Geometry check sheet. Reference: the model listing, model coordinates, mm. Face numbers are marked on the shaded views. A direction names the side the tool comes from. Round coordinates to 2 decimals unless told otherwise and drop trailing zeros. Loops run counter-clockwise (first coordinate to the right, second up) from the corner with the lowest first, then second, coordinate; pieces in that order, holes last. Notation, with made-up numbers: (-12.75, 62.5) -> (37.25, 62.5) arc R23 cw to (37.25, 98.5) -> close; hole circle Ø2 at (15, 18). An arc over 180 degrees is marked (long way). Use one line per item in the form item = value.
from build123d import *

# Parameters (mm, degrees)
SKETCH_1_W          = 39.5
SKETCH_1_H          = 34.04
EXTRUDE_1_DEPTH     = 2
SKETCH_2_R          = 1.25
CUT_EXTRUDE_1_DEPTH = 2
SKETCH_3_R          = 12.5
EXTRUDE_2_DEPTH     = 5
FILLET_1_R          = 1
SKETCH_4_W          = 8
SKETCH_4_H          = 8.5
SKETCH_4_H_2        = 12
EXTRUDE_3_DEPTH     = 5
SKETCH_5_R          = 1
CUT_EXTRUDE_2_DEPTH = 5


with BuildPart() as part:
    # 草图1 → 凸台-拉伸1 (new body)
    with BuildSketch(Plane.XY):
        Rectangle(SKETCH_1_W, SKETCH_1_H)
    extrude(amount=EXTRUDE_1_DEPTH)

    # 草图2 → 切除-拉伸1 (cut)
    with BuildSketch(Plane.XY.offset(2)):
        with Locations((-16.95, 14.225)):
            Circle(SKETCH_2_R)
        with Locations((-16.95, -14.225)):
            Circle(SKETCH_2_R)
        with Locations((8.07, 14.225)):
            Circle(SKETCH_2_R)
        with Locations((8.07, -14.225)):
            Circle(SKETCH_2_R)
    extrude(amount=-CUT_EXTRUDE_1_DEPTH, mode=Mode.SUBTRACT)

    # 草图3 → 凸台-拉伸2 (add)
    with BuildSketch(Plane.XY.offset(2)):
        with Locations(Location((-4.44, 0, 0), (0, 0, 180))):
            Circle(SKETCH_3_R)
    extrude(amount=EXTRUDE_2_DEPTH)

    # 圆角1
    fillet_1_edges = [part.edges().sort_by_distance(p)[0] for p in [
        (19.75, -17.02, 1),
        (-19.75, -17.02, 1),
        (-19.75, 17.02, 1),
        (19.75, 17.02, 1),
    ]]
    fillet(fillet_1_edges, radius=FILLET_1_R)

    # 草图4 → 凸台-拉伸3 (add)
    with BuildSketch(Plane.XY.offset(2)):
        with Locations((15.75, 8.25)):
            Rectangle(SKETCH_4_W, SKETCH_4_H)
        with Locations((15.75, -6.5)):
            Rectangle(SKETCH_4_W, SKETCH_4_H_2)
    extrude(amount=EXTRUDE_3_DEPTH)

    # 草图5 → 切除-拉伸2 (cut)
    with BuildSketch(Plane.XY.offset(7)):
        with Locations((-6.44, 6.464101615)):
            Circle(SKETCH_5_R)
        with Locations((-2.44, 6.464101615)):
            Circle(SKETCH_5_R)
        with Locations((-4.44, 3)):
            Circle(SKETCH_5_R)
        with Locations(Location((-4.44, -3, 0), (0, 0, 180))):
            Circle(SKETCH_5_R)
        with Locations(Location((-2.44, -6.464101615, 0), (0, 0, 180))):
            Circle(SKETCH_5_R)
        with Locations(Location((-6.44, -6.464101615, 0), (0, 0, 180))):
            Circle(SKETCH_5_R)
    extrude(amount=-CUT_EXTRUDE_2_DEPTH, mode=Mode.SUBTRACT)


solid = part.part
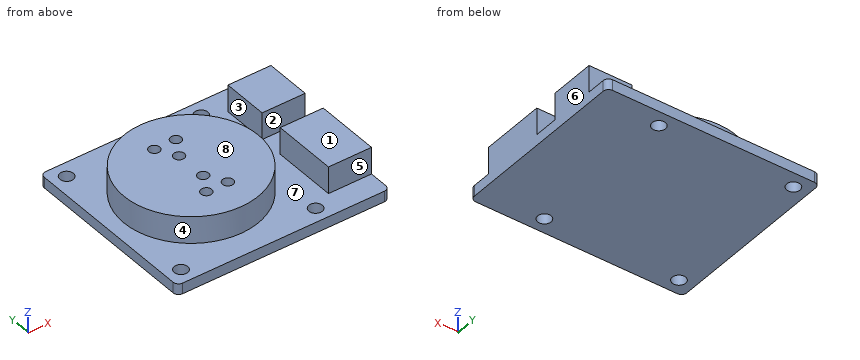
1. Tool access check on the marked faces 1, 2, 3, 4 and 5. Record the directions out of +Z, -Z, +X, -X, +Y, -Y that give a thin tool (end or side, any length) a straight path to the whole face; none if there is none.
Return value:
face_1 = +Z, +X, -X, +Y, -Y
face_2 = +Z, +X
face_3 = +Z, +Y, -Y
face_4 = +Z
face_5 = +Z, +X, -X, -Y
2. Section check A-A (z = 2.5). Count the separate pieces of the cut face and the enclosed holes in it, then the cut area to 3 significant figures.
Return value:
separate_pieces = 3
enclosed_holes = 6
area = 636 mm2
3. Section check D-D (z = 0.5). Record the boundary of the cut face in (x, y) (3 decimals).
Return value:
outline = (-19.75, -16.02) arc R1 ccw to (-18.75, -17.02) -> (18.75, -17.02) arc R1 ccw to (19.75, -16.02) -> (19.75, 16.02) arc R1 ccw to (18.75, 17.02) -> (-18.75, 17.02) arc R1 ccw to (-19.75, 16.02) -> close; hole circle Ø2.5 at (-16.95, -14.225); hole circle Ø2.5 at (-16.95, 14.225); hole circle Ø2.5 at (8.07, -14.225); hole circle Ø2.5 at (8.07, 14.225)
4. Material ranges on line 1 along Y through (x, z) = (-16.95, 0.7) (3 decimals); line 2 along Y through (x, z) = (-2.44, 5.2); line 3 along X through (y, z) = (-3, 3.45), recorded low to high.
Return value:
line_1 = -17.02 to -15.475, -12.975 to 12.975, 15.475 to 17.02
line_2 = -12.34 to -7.46, -5.46 to 5.46, 7.46 to 12.34
line_3 = -16.57 to -5.44, -3.44 to 7.69, 11.75 to 19.75
5. Section check B-B (y = -1). Record the boundary of the cut face in (x, z).
Return value:
outline = (-19.75, 0) -> (19.75, 0) -> (19.75, 7) -> (11.75, 7) -> (11.75, 2) -> (8.02, 2) -> (8.02, 7) -> (-16.9, 7) -> (-16.9, 2) -> (-19.75, 2) -> close
6. Mould release check, pull along X, two halves, no side actions. Record for the marked faces 6, 7 and 8: released by +X, released by -X, zero draft, split by the parting line, or undercut.
Return value:
face_6 = released by +X
face_7 = undercut
face_8 = zero draft
7. Gauge pin test, flat ends, axial feed: pin 1 (2.5 mm diameter, centred on x = 17, z = 4, fed in from -Y); pin 2 (1 mm diameter, centred on x = -6.5, y = -6.5, fed in from +Z). Record the tip position at first contact, or that the pin passes through.
Return value:
pin_1 = -12.5
pin_2 = 2
8. Section check C-C (x = -2.44). Record the boundary of the cut face in (y, z), then the cut area to 3 significant figures.
Return value:
outline = (-17.02, 0) -> (17.02, 0) -> (17.02, 2) -> (12.34, 2) -> (12.34, 7) -> (7.46, 7) -> (7.46, 2) -> (5.46, 2) -> (5.46, 7) -> (-5.46, 7) -> (-5.46, 2) -> (-7.46, 2) -> (-7.46, 7) -> (-12.34, 7) -> (-12.34, 2) -> (-17.02, 2) -> close
area = 171 mm2
